CAD build for the part. Positions are in the model's coordinates, mm. A direction names the side the tool comes from. Give positions to 0.01 mm unless a question says otherwise; leave off trailing zeros. Order: outer loops, then holes, each group sorted by start corner. A loop starts at its lowest first (then second) coordinate and runs counter-clockwise, first axis right, second up. Notation, with made-up numbers: (40, -33) -> (77, -33) arc R3 ccw to (77, -28) -> close; hole circle Ø7 at (49, 44.25). An arc over 180 degrees is marked (long way). Answer as CSV lines item,"result".
```python
from build123d import *

# Parameters (mm, degrees)
SKETCH1_R           = 3.25
SKETCH1_R_2         = 20
BOSS_EXTRUDE1_DEPTH = 19.5
SKETCH2_R           = 31.25
CUT_EXTRUDE1_DEPTH  = 16.5
SKETCH3_R           = 5.25
CUT_EXTRUDE2_DEPTH  = 10
SKETCH4_R           = 1.25
CUT_EXTRUDE3_DEPTH  = 80
SKETCH5_R           = 1.25
CUT_EXTRUDE4_DEPTH  = 80


with BuildPart() as part:
    # Sketch1 → Boss-Extrude1 (new body)
    with BuildSketch(Plane(origin=(0, 0, 0), x_dir=(1, 0, 0), z_dir=(0, 1, 0))):
        with BuildLine():
            Line((-21.388284323, 40), (-33.157842357, 42.785014786))
            ThreePointArc((-33.157842357, 42.785014786), (-40.656854249, 40.656854249), (-42.785014786, 33.157842357))
            Line((-42.785014786, 33.157842357), (-40, 21.388284323))
            Line((-40, 21.388284323), (-40, -21.388284323))
            Line((-40, -21.388284323), (-42.785014786, -33.157842357))
            ThreePointArc((-42.785014786, -33.157842357), (-40.656854249, -40.656854249), (-33.157842357, -42.785014786))
            Line((-33.157842357, -42.785014786), (-21.388284323, -40))
            Line((-21.388284323, -40), (21.388284323, -40))
            Line((21.388284323, -40), (33.157842357, -42.785014786))
            ThreePointArc((33.157842357, -42.785014786), (40.656854249, -40.656854249), (42.785014786, -33.157842357))
            Line((42.785014786, -33.157842357), (40, -21.388284323))
            Line((40, -21.388284323), (40, 21.388284323))
            Line((40, 21.388284323), (42.785014786, 33.157842357))
            ThreePointArc((42.785014786, 33.157842357), (40.656854249, 40.656854249), (33.157842357, 42.785014786))
            Line((33.157842357, 42.785014786), (21.388284323, 40))
            Line((21.388284323, 40), (-21.388284323, 40))
        make_face()
        with Locations((35, 35)):
            Circle(SKETCH1_R, mode=Mode.SUBTRACT)
        with Locations((-35, -35)):
            Circle(SKETCH1_R, mode=Mode.SUBTRACT)
        with Locations((35, -35)):
            Circle(SKETCH1_R, mode=Mode.SUBTRACT)
        with Locations((-35, 35)):
            Circle(SKETCH1_R, mode=Mode.SUBTRACT)
        Circle(SKETCH1_R_2, mode=Mode.SUBTRACT)
    extrude(amount=BOSS_EXTRUDE1_DEPTH)

    # Sketch2 → Cut-Extrude1 (cut)
    with BuildSketch(Plane(origin=(0, 19.5, 0), x_dir=(1, 0, 0), z_dir=(0, 1, 0))):
        Circle(SKETCH2_R)
    extrude(amount=-CUT_EXTRUDE1_DEPTH, mode=Mode.SUBTRACT)

    # Sketch3 → Cut-Extrude2 (cut)
    with BuildSketch(Plane.XZ):
        with Locations((-35, 35)):
            Circle(SKETCH3_R)
        with Locations((35, 35)):
            Circle(SKETCH3_R)
        with Locations((35, -35)):
            Circle(SKETCH3_R)
        with Locations((-35, -35)):
            Circle(SKETCH3_R)
    extrude(amount=-CUT_EXTRUDE2_DEPTH, mode=Mode.SUBTRACT)

    # Sketch4 → Cut-Extrude3 (cut)
    with BuildSketch(Plane.XY.offset(40)):
        with Locations((0, 9.75)):
            Circle(SKETCH4_R)
    extrude(amount=-CUT_EXTRUDE3_DEPTH, mode=Mode.SUBTRACT)

    # Sketch5 → Cut-Extrude4 (cut)
    with BuildSketch(Plane(origin=(40, 0, 0), x_dir=(0, 0, -1), z_dir=(1, 0, 0))):
        with Locations((0, 9.75)):
            Circle(SKETCH5_R)
    extrude(amount=-CUT_EXTRUDE4_DEPTH, mode=Mode.SUBTRACT)


solid = part.part
```
1) Band-saw the part on A-A, the plane x = -35. Write the cut outline in (y, z), then the cut area to 3 significant figures.
Data:
outline,"(0, -43) -> (19.5, -43) -> (19.5, -38.25) -> (10, -38.25) -> (10, -40.25) -> (0, -40.25) -> close; (0, -29.75) -> (10, -29.75) -> (10, -31.75) -> (19.5, -31.75) -> (19.5, 31.75) -> (10, 31.75) -> (10, 29.75) -> (0, 29.75) -> close; (0, 40.25) -> (10, 40.25) -> (10, 38.25) -> (19.5, 38.25) -> (19.5, 43) -> (0, 43) -> close; hole circle Ø2.5 at (9.75, 0)"
area,"1,340 mm2"
2) Which spindle directions (+Z, -Z, +X, -X, +Y, -Y) get a long thin tool onto all of the face, cutting with end or side? Do faces 3 (the cylindrical face through (36.5, 14.683, -32.117)), 4 (the flat face through (40, 12, 0)), 5 (the flat face through (-0.4, 3, 20.4)), 6 (the flat face through (-41.412, 9.614, -27.355)), 7 (the cylindrical face through (31.13, 4.93, 38.55)). Say none if no direction does.
Data:
face 3,"+Y, -Y"
face 4,"+X, +Y, -Y"
face 5,"+Y"
face 6,"-X, +Y, -Y"
face 7,"-Y"
3) Wall check: line 1 along Z through (x, y) = (35, 14.5); line 2 along Z through (x, y) = (35, 6.25). Give the ranges that are in metal, low to high. Write a range as [from, to].
Data:
line 1,"z = [-43, -38.25], [-31.75, 31.75], [38.25, 43]"
line 2,"z = [-43, -40.25], [-29.75, 29.75], [40.25, 43]"
4) Band-saw the part on B-B, the plane z = -35. Write the cut outline in (x, y).
Data:
outline,"(-43, 0) -> (-40.25, 0) -> (-40.25, 10) -> (-38.25, 10) -> (-38.25, 19.5) -> (-43, 19.5) -> close; (-31.75, 10) -> (-29.75, 10) -> (-29.75, 0) -> (29.75, 0) -> (29.75, 10) -> (31.75, 10) -> (31.75, 19.5) -> (-31.75, 19.5) -> close; (38.25, 10) -> (40.25, 10) -> (40.25, 0) -> (43, 0) -> (43, 19.5) -> (38.25, 19.5) -> close; hole circle Ø2.5 at (0, 9.75)"
5) Band-saw the part on C-C, the plane z = 0. Write the cut outline in (x, y), then the cut area to 3 significant figures.
Data:
outline,"(-40, 0) -> (-20, 0) -> (-20, 3) -> (-31.25, 3) -> (-31.25, 8.5) -> (-40, 8.5) -> close; (-40, 11) -> (-31.25, 11) -> (-31.25, 19.5) -> (-40, 19.5) -> close; (20, 0) -> (40, 0) -> (40, 8.5) -> (31.25, 8.5) -> (31.25, 3) -> (20, 3) -> close; (31.25, 11) -> (40, 11) -> (40, 19.5) -> (31.25, 19.5) -> close"
area,"365 mm2"
6) Pin check, flat tips, straight feed: P1, Ø5, axis at y = 17, z = -9.5, coming from the +X side; P2, Ø2, axis at x = 0, y = 9.75, coming from the +Z side; P3, Ø1, axis at y = 6.5, z = -30, coming from the -X side; P4, Ø8, axis at x = -5.5, y = 2.5, coming from the -Z side. Stop position of each tip, or through.
Data:
P1,"stops at x = 40"
P2,"passes through"
P3,"stops at x = -42.16"
P4,"stops at z = -40"
7) Band-saw the part on D-D, the plane y = 4.5. Write the cut outline in (x, z).
Data:
outline,"(-42.79, -33.16) arc R8 ccw to (-33.16, -42.79) -> (-21.39, -40) -> (21.39, -40) -> (33.16, -42.79) arc R8 ccw to (42.79, -33.16) -> (40, -21.39) -> (40, 21.39) -> (42.79, 33.16) arc R8 ccw to (33.16, 42.79) -> (21.39, 40) -> (-21.39, 40) -> (-33.16, 42.79) arc R8 ccw to (-42.79, 33.16) -> (-40, 21.39) -> (-40, -21.39) -> close; hole circle Ø10.5 at (-35, -35); hole circle Ø10.5 at (-35, 35); hole circle Ø62.5 at (0, 0); hole circle Ø10.5 at (35, -35); hole circle Ø10.5 at (35, 35)"
8) Pull direction Z, two halves, no side cores. Call faces 1 (the flat face through (-35.1, 10, 31.6)), 2 (the flat face through (-27.355, 9.614, 41.412)): pulls with the +Z half, pulls with the -Z half, needs draft (parallel to the pull), parting line crosses it, or undercut.
Data:
face 1,"undercut"
face 2,"pulls with the +Z half"
